Can you work these out from the drawing? Everything is in mm from the part's minimum corner. Coordinates: 2 decimals unless noted, no trailing zeros. Loops run counter-clockwise (first coordinate to the right, second up) from the corner with the lowest first, then second, coordinate; pieces in that order, holes last. Notation, with made-up numbers: (54.5, 33.25) - (84.5, 33.25) arc R34 cw to (84.5, 65.25) - close; hole circle Ø4 at (-1.75, 37). An arc over 180 degrees is marked (long way). One line per question, with ' | ' between items. Start each with the question number.
1. I want a section at B-B, the plane y = 1.5. Write out the boundary of the cut face in (x, z).
2. I'm going to push flat-ended pins straight in: P1, Ø3.5, axis at x = 8, z = 19, coming from the +Y side; P2, Ø3, axis at y = 2, z = 14.5, coming from the -X side. Where does each tip first touch, or does it pass through?
3. I want a section at A-A, the plane x = 8. Write out the boundary of the cut face in (y, z).
4. Please list where these lines run through material, in increasing order: L1, parallel to X at y = 8.5, z = 19.5; L2, parallel to X at y = 11, z = 4; L3, parallel to X at y = 10, z = 16.25. Write a range as [from, to].
5. We'd pull the mould along X, two halves only. Please class the marked faces 1, 2, 3 and 4: pulls with the +X half, pulls with the -X half, needs draft (parallel to the pull), parting line crosses it, or undercut.
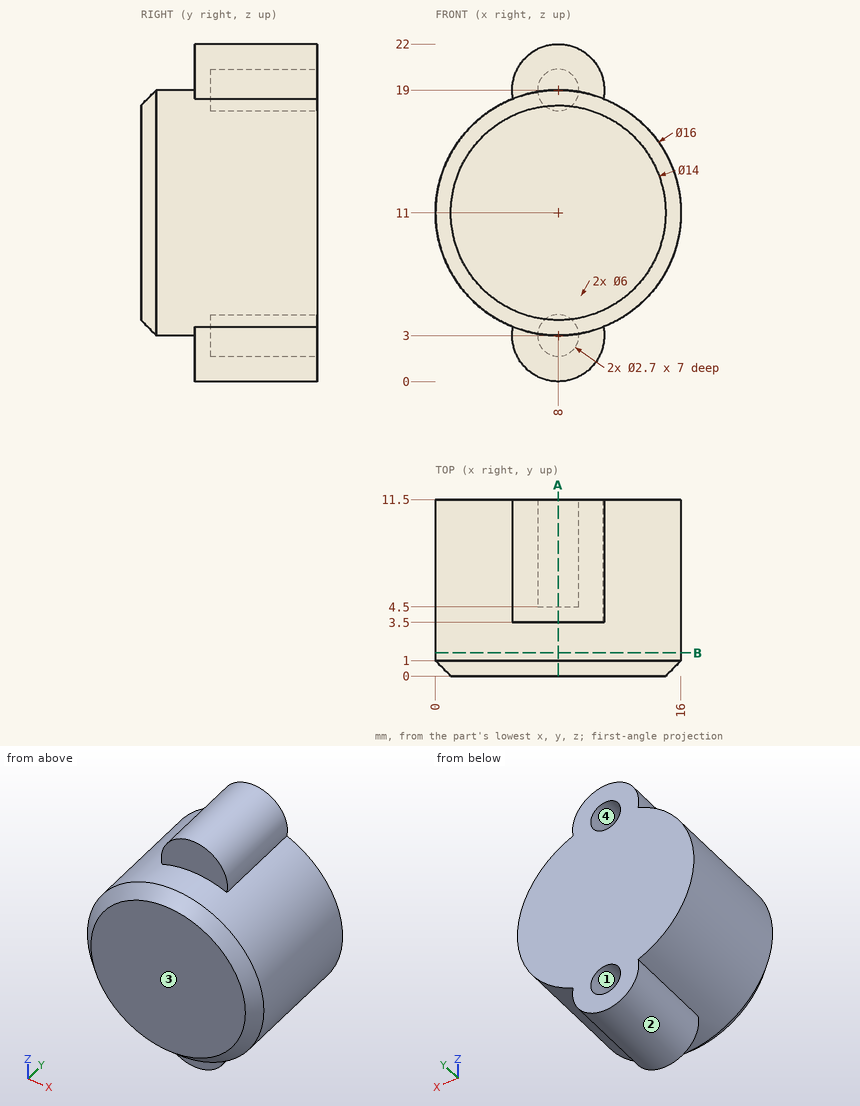
Results are:
1) outline: circle Ø16 at (8, 11)
2) P1: stops at y = 11.5 | P2: stops at x = 0.25
3) outline: (0, 4) - (1, 3) - (3.5, 3) - (3.5, 0) - (11.5, 0) - (11.5, 1.65) - (4.5, 1.65) - (4.5, 4.35) - (11.5, 4.35) - (11.5, 17.65) - (4.5, 17.65) - (4.5, 20.35) - (11.5, 20.35) - (11.5, 22) - (3.5, 22) - (3.5, 19) - (1, 19) - (0, 18) - close
4) L1: x = [5.04, 6.75], [9.25, 10.96] | L2: x = [4.13, 7.09], [8.91, 11.87] | L3: x = [1.96, 14.04]
5) face 1: undercut | face 2: parting line crosses it | face 3: needs draft | face 4: undercut
